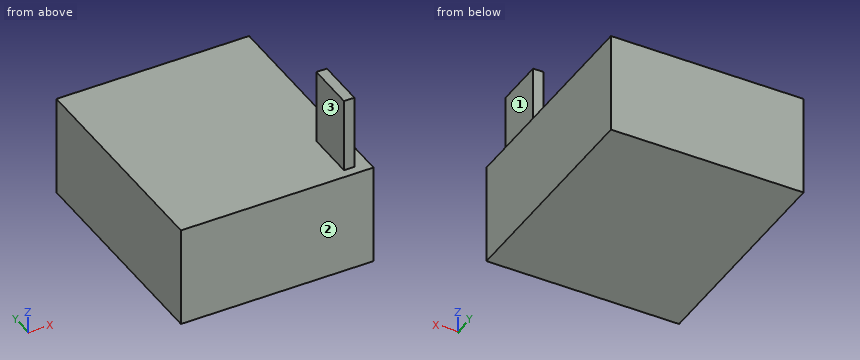
from build123d import *

# Parameters (mm, degrees)
F0_W     = 65.53819
F0_H     = 34.391328
F1_DEPTH = 76.2
F2_W     = 3.561789
F2_H     = 16.879741
F3_DEPTH = 25.4


with BuildPart() as f1:
    # F0 (on Front) → F1 (new body)
    with BuildSketch(Plane.XZ):
        Rectangle(F0_W, F0_H)
    extrude(amount=F1_DEPTH)

    # F2 (on face) → F3 (join)
    with BuildSketch(Plane.XY.offset(17.195664)):
        with Locations((26.195521, -64.690722)):
            Rectangle(F2_W, F2_H)
    extrude(amount=F3_DEPTH)


solid = f1.part
Geometry: final body of the model. Coordinates: model frame, mm. Face numbers are marked on the shaded views. A direction names the side the tool comes from. Coordinates: 2 decimals unless noted, no trailing zeros. Order: outer loops, then holes, each group sorted by start corner. A loop starts at its lowest first (then second) coordinate and runs counter-clockwise, first axis right, second up.
1) Section A-A (y = -72). Return loops of the section in (x, z), then the cut area to 3 significant figures.
Result sheet:
outline: (-32.77, -17.2) - (32.77, -17.2) - (32.77, 17.2) - (27.98, 17.2) - (27.98, 42.6) - (24.41, 42.6) - (24.41, 17.2) - (-32.77, 17.2) - close
area: 2,340 mm2
2) Section C-C (z = 34). Return loops of the section in (x, y).
Result sheet:
outline: (24.41, -73.13) - (27.98, -73.13) - (27.98, -56.25) - (24.41, -56.25) - close
3) Set-up query: the marked faces 1, 2 and 3. Return all of +Z, -Z, +X, -X, +Y, -Y with unobstructed straight access to the full face (end or side cutting, diameter ignored); none if empty.
Result sheet:
face 1: +Z, +X, +Y, -Y
face 2: +Z, -Z, +X, -X, -Y
face 3: +Z, -X, +Y, -Y
4) First-contact query: P1, Ø4, axis at x = 25.5, z = 32.5, coming from the -Y side; P2, Ø18.5, axis at y = -62, z = 34.5, coming from the +X side; P3, Ø5, axis at x = -13.5, y = -15, coming from the +Z side. Flat tips, straight axial feed; report the tip coordinate or a pass-through.
Result sheet:
P1: stops at y = -73.13
P2: stops at x = 27.98
P3: stops at z = 17.2
5) Section B-B (x = -5.5). Return loops of the section in (y, z), then the cut area to 3 significant figures.
Result sheet:
outline: (-76.2, -17.2) - (0, -17.2) - (0, 17.2) - (-76.2, 17.2) - close
area: 2,620 mm2
6) Ray query, probe 1 along Z at (x, y) = (6.5, -20); probe 2 along Y at (x, z) = (26, 18); probe 3 along X at (y, z) = (-63, 32). Return the intervals inside material, ascending.
Result sheet:
probe 1: z = -17.2 to 17.2
probe 2: y = -73.13 to -56.25
probe 3: x = 24.41 to 27.98
